Part model, mm, in its own coordinate system. Coordinates: 2 decimals unless noted, no trailing zeros. Loops run counter-clockwise (first coordinate to the right, second up) from the corner with the lowest first, then second, coordinate; pieces in that order, holes last. Notation, with made-up numbers: (-26, -37.5) -> (25, -37.5) arc R29 ccw to (25, -4.5) -> close; hole circle Ø11 at (25, 76.25). An arc over 180 degrees is marked (long way). One line per item, written item: value. Start each with the question number.
from build123d import *

# Parameters (mm, degrees)
F1_W     = 330.2
F1_H     = 228.6
F2_DEPTH = 10
F3_SIZE  = 9.99999


# Not quite as in the source:
# - a fillet or chamfer is up to 0.001 mm smaller than in the source, because OpenCascade refuses the exact size


with BuildPart() as f2:
    # F1 (on face) → F2 (new body)
    with BuildSketch(Plane.XZ):
        Rectangle(F1_W, F1_H)
    extrude(amount=F2_DEPTH)

    # F3 (size 10 in the source; OpenCascade refuses exactly that, so slightly less here)
    f3_edges = [f2.edges().sort_by_distance(p)[0] for p in [
        (0, 0, 114.3),
        (165.1, 0, 0),
        (-165.1, 0, 0),
        (0, 0, -114.3),
    ]]
    chamfer(f3_edges, length=F3_SIZE)


solid = f2.part
1) Probe line 1 (X direction, y = -8, z = -95); line 2 (X direction, y = -4, z = 60.5); line 3 (Z direction, x = 144.5, y = -3.75). List the from-to ranges inside material, lowest first. Write a range as from..to.
2) Pin check, flat tips, straight feed: pin 1 Ø4 at (x, y) = (0, -8.5) entering from +Z; pin 2 Ø1 at (x, y) = (122.5, -6) entering from -Z; pin 3 Ø4 at (y, z) = (-3.5, 75.5) entering from -X; pin 4 Ø1.5 at (y, z) = (-7, -88) entering from -X. Stop position of each tip, or through.
3) Slice it at C-C (y = -5.25). Give the cut face in (x, z), then the cut area to 3 significant figures.
Check sheet entries:
1. line 1: x = -163.1..163.1
1. line 2: x = -159.1..159.1
1. line 3: z = -108.05..108.05
2. pin 1: stops at z = 114.3
2. pin 2: stops at z = -110.8
2. pin 3: stops at x = -160.6
2. pin 4: stops at x = -162.85
3. outline: (-160.35, -109.55) -> (160.35, -109.55) -> (160.35, 109.55) -> (-160.35, 109.55) -> close
3. area: 70,300 mm^2
